from build123d import *

# Parameters (mm, degrees)
SKETCH1_R           = 41.075
SKETCH1_R_2         = 3.175
SKETCH1_R_3         = 18.796
BOSS_EXTRUDE2_DEPTH = 6.35


with BuildPart() as part:
    # Sketch1 → Boss-Extrude2 (new body)
    with BuildSketch(Plane(origin=(0, 0, 0), x_dir=(1, 0, 0), z_dir=(0, 1, 0))):
        Circle(SKETCH1_R)
        with Locations((0, 34.725)):
            Circle(SKETCH1_R_2, mode=Mode.SUBTRACT)
        with Locations((34.725, 0)):
            Circle(SKETCH1_R_2, mode=Mode.SUBTRACT)
        with Locations((-34.725, 0)):
            Circle(SKETCH1_R_2, mode=Mode.SUBTRACT)
        Circle(SKETCH1_R_3, mode=Mode.SUBTRACT)
    extrude(amount=BOSS_EXTRUDE2_DEPTH)


solid = part.part
Could you check a few things on this model? Use its own coordinates, in mm. Round coordinates to 2 decimals unless told otherwise and drop trailing zeros. Write each loop counter-clockwise with the first axis right and the second up, starting at its lowest first coordinate (ties: lowest second). Pieces come first, ordered by that corner, then holes. Notation, with made-up numbers: (38.5, -0.5) -> (43.5, -0.5) arc R20 ccw to (43.5, 23.5) -> close; hole circle Ø6 at (26, 70.5). An arc over 180 degrees is marked (long way). Use a Markdown table: item, result.
1. If we section it at D-D (z = 14): List the corners of the cut face in (x, y) for me.
Answer key:
| item | result |
|---|---|
| outline | (-38.62, 0) -> (-12.54, 0) -> (-12.54, 6.35) -> (-38.62, 6.35) -> close; (12.54, 0) -> (38.62, 0) -> (38.62, 6.35) -> (12.54, 6.35) -> close |
2. If we section it at C-C (x = 10): List the corners of the cut face in (y, z) for me, then the cut area to 3 significant figures.
Answer key:
| item | result |
|---|---|
| outline | (0, -39.84) -> (6.35, -39.84) -> (6.35, -15.92) -> (0, -15.92) -> close; (0, 15.92) -> (6.35, 15.92) -> (6.35, 39.84) -> (0, 39.84) -> close |
| area | 304 mm^2 |
3. Please list where these lines run through material, in increasing order: probe 1 along Z at (x, y) = (0, 2) (3 decimals); probe 2 along X at (y, z) = (1, -2); probe 3 along Z at (x, y) = (-2.5, 5).
Answer key:
| item | result |
|---|---|
| probe 1 | z = -41.075 to -37.9, -31.55 to -18.796, 18.796 to 41.075 |
| probe 2 | x = -41.03 to -37.19, -32.26 to -18.69, 18.69 to 32.26, 37.19 to 41.03 |
| probe 3 | z = -41 to -36.68, -32.77 to -18.63, 18.63 to 41 |
4. For pin 1 Ø1.5 at (x, y) = (2, 4) entering from +Z; pin 2 Ø1 at (x, y) = (-3, 1) entering from -Z; pin 3 Ø1 at (x, y) = (-8.5, 0.5) entering from -Z; pin 4 Ø2 at (x, z) = (-26.5, -8) entering from -Y, each with a flat end and sliding along its axis, tell me the tip position at first contact or that it passes through.
Answer key:
| item | result |
|---|---|
| pin 1 | stops at z = 41.06 |
| pin 2 | stops at z = -41 |
| pin 3 | stops at z = -40.29 |
| pin 4 | stops at y = 0 |
5. If we section it at A-A (x = 0): List the corners of the cut face in (y, z) for me (3 decimals).
Answer key:
| item | result |
|---|---|
| outline | (0, -41.075) -> (6.35, -41.075) -> (6.35, -37.9) -> (0, -37.9) -> close; (0, -31.55) -> (6.35, -31.55) -> (6.35, -18.796) -> (0, -18.796) -> close; (0, 18.796) -> (6.35, 18.796) -> (6.35, 41.075) -> (0, 41.075) -> close |
6. We'd pull the mould along X, two halves only. Please class faces 1 (the face through (32.385, 3.131, -2.146)), 2 (the face through (39.178, 3.131, -12.338)), 3 (the face through (1.71, 3.13, -37.4)), 4 (the face through (9, 0, 18)): +X half, -X half, draft (parallel to the pull), parting line (faces both ways), or undercut.
Answer key:
| item | result |
|---|---|
| face 1 | undercut |
| face 2 | parting line |
| face 3 | undercut |
| face 4 | draft |
7. If we section it at B-B (z = 0): List the corners of the cut face in (x, y) for me (3 decimals).
Answer key:
| item | result |
|---|---|
| outline | (-41.075, 0) -> (-37.9, 0) -> (-37.9, 6.35) -> (-41.075, 6.35) -> close; (-31.55, 0) -> (-18.796, 0) -> (-18.796, 6.35) -> (-31.55, 6.35) -> close; (18.796, 0) -> (31.55, 0) -> (31.55, 6.35) -> (18.796, 6.35) -> close; (37.9, 0) -> (41.075, 0) -> (41.075, 6.35) -> (37.9, 6.35) -> close |
